```python
from build123d import *

# Parameters (mm, degrees)
F1_DEPTH = 2
F3_DEPTH = 5.4
F4_R     = 2.5
F5_DEPTH = 2
F6_R     = 1.25
F7_DEPTH = 25


with BuildPart() as f1:
    # F0 (on Top) → F1 (new body)
    with BuildSketch(Plane.XY):
        with BuildLine():
            Line((-7.5, 10), (-7.5, 0))
            ThreePointArc((-7.5, 0), (0, -7.5), (7.5, 0))
            Line((7.5, 0), (7.5, 10))
            Line((7.5, 10), (1.40202, 26.033235))
            ThreePointArc((1.40202, 26.033235), (0, 27), (-1.40202, 26.033235))
            Line((-1.40202, 26.033235), (-7.5, 10))
        make_face()
    extrude(amount=F1_DEPTH)

    # F2 (on face) → F3 (join)
    with BuildSketch(Plane.XY.offset(2)):
        with BuildLine():
            Line((-7.5, 10), (-7.5, 0))
            ThreePointArc((-7.5, 0), (0, -7.5), (7.5, 0))
            Line((7.5, 0), (7.5, 10))
            Line((7.5, 10), (5, 7.5))
            Line((5, 7.5), (5, 0))
            ThreePointArc((5, 0), (0, -5), (-5, 0))
            Line((-5, 0), (-5, 7.5))
            Line((-5, 7.5), (-7.5, 10))
        make_face()
    extrude(amount=F3_DEPTH)

    # F4 (on face) → F5 (join)
    with BuildSketch(Plane(origin=(0, 0, 0), x_dir=(1, 0, 0), z_dir=(0, 0, -1))):
        with Locations((0, -16)):
            Circle(F4_R)
    extrude(amount=F5_DEPTH)

    # F6 (on face) → F7 (cut)
    with BuildSketch(Plane(origin=(0, 0, -2), x_dir=(1, 0, 0), z_dir=(0, 0, -1))):
        with Locations((0, -16)):
            Circle(F6_R)
    extrude(amount=-F7_DEPTH, mode=Mode.SUBTRACT)


solid = f1.part
```
Design review of the part built by this model. Coordinates are the model's own, in mm. A direction names the side the tool comes from. Give positions to 0.01 mm unless a question says otherwise; leave off trailing zeros. Write each loop counter-clockwise with the first axis right and the second up, starting at its lowest first coordinate (ties: lowest second). Pieces come first, ordered by that corner, then holes. Notation, with made-up numbers: (71.25, 84.25) - (99.25, 84.25) arc R23 ccw to (99.25, 123.25) - close; hole circle Ø2 at (45, -11.75). An arc over 180 degrees is marked (long way). Return JSON: item names as keys, results as strings. Group by question number.
(1) We need section D-D, the plane z = 1. Give the boundary of the cut face in (x, y).
(2) Machinability: for faces 4 (the cylindrical face through (-0.54, 18.44, -0.99)), 5 (the cylindrical face through (0, -5, 5)), 6 (the flat face through (-4.41, 18.13, 0.99)), which of the approach directions +Z, -Z, +X, -X, +Y, -Y give a long, thin tool a straight path to every point of the face, cutting with its end or side? Answer none if there is none.
(3) To check wall thickness, follow probe 1 along X at (y, z) = (3, 4.5); probe 2 along Y at (x, z) = (0, -0.95); probe 3 along Y at (x, z) = (0, 1.2). State the ranges of each line that lie inside material, in increasing order.
(4) Insertion check: pin 1 (5 mm diameter, centred on x = 1, y = 6.5, fed in from -Z); pin 2 (4 mm diameter, centred on x = 3.5, z = 3, fed in from -Y); pin 3 (5 mm diameter, centred on x = -5.5, y = 21.5, fed in from +Z); pin 4 (1.5 mm diameter, centred on x = 0, y = 16, fed in from +Z). Each pin has a flat end and moves straight along its axis. Give the tip position at first contact, or say it passes through.
(5) We need section A-A, the plane y = 16. Give the boundary of the cut face in (x, z).
(6) Mouldability with a two-part tool opening along X and no side actions: class faces 1 (the flat face through (0, 11, 2)), 2 (the flat face through (7.5, 5, 4)), 3 (the cylindrical face through (0, 27, 1)) as +X half, -X half, draft (parallel to the pull), parting line (faces both ways), or undercut.
(7) We need section C-C, the plane x = 0.25. Give the boundary of the cut face in (y, z).
(8) We need section B-B, the plane z = 3.75. Give the boundary of the cut face in (x, y).
Reported:
{
 "1": {"outline": "(-7.5, 0) arc R7.5 ccw to (7.5, 0) - (7.5, 10) - (1.4, 26.03) arc R1.5 ccw to (-1.4, 26.03) - (-7.5, 10) - close; hole circle Ø2.5 at (0, 16)"},
 "2": {"face 4": "-Z", "face 5": "+Z, +Y", "face 6": "+Z, -Z, -X, +Y"},
 "3": {"probe 1": "x = -7.5 to -5, 5 to 7.5", "probe 2": "y = 13.5 to 14.75, 17.25 to 18.5", "probe 3": "y = -7.5 to 14.75, 17.25 to 27"},
 "4": {"pin 1": "stops at z = 0", "pin 2": "stops at y = -7.35", "pin 3": "stops at z = 2", "pin 4": "passes through"},
 "5": {"outline": "(-5.22, 0) - (-2.5, 0) - (-2.5, -2) - (-1.25, -2) - (-1.25, 2) - (-5.22, 2) - close; (1.25, -2) - (2.5, -2) - (2.5, 0) - (5.22, 0) - (5.22, 2) - (1.25, 2) - close"},
 "6": {"face 1": "undercut", "face 2": "+X half", "face 3": "parting line"},
 "7": {"outline": "(-7.5, 0) - (13.51, 0) - (13.51, -2) - (14.78, -2) - (14.78, 2) - (-4.99, 2) - (-4.99, 7.4) - (-7.5, 7.4) - close; (17.22, -2) - (18.49, -2) - (18.49, 0) - (26.98, 0) - (26.98, 2) - (17.22, 2) - close"},
 "8": {"outline": "(-7.5, 0) arc R7.5 ccw to (7.5, 0) - (7.5, 10) - (5, 7.5) - (5, 0) arc R5 cw to (-5, 0) - (-5, 7.5) - (-7.5, 10) - close"}
}
